The drawing under review shows one solid part. Ordinate dimensions are in mm from its lowest x, y, z. A direction names the side the tool comes from. Give positions to 0.01 mm unless a question says otherwise; leave off trailing zeros. Loops run counter-clockwise (first coordinate to the right, second up) from the corner with the lowest first, then second, coordinate; pieces in that order, holes last. Notation, with made-up numbers: (-4, 57.25) - (42, 57.25) arc R28 ccw to (42, 91.25) - close; hole circle Ø4 at (-10.5, -32.5). An arc over 180 degrees is marked (long way). Return JSON: item names as keys, results as strings. Group by question number.
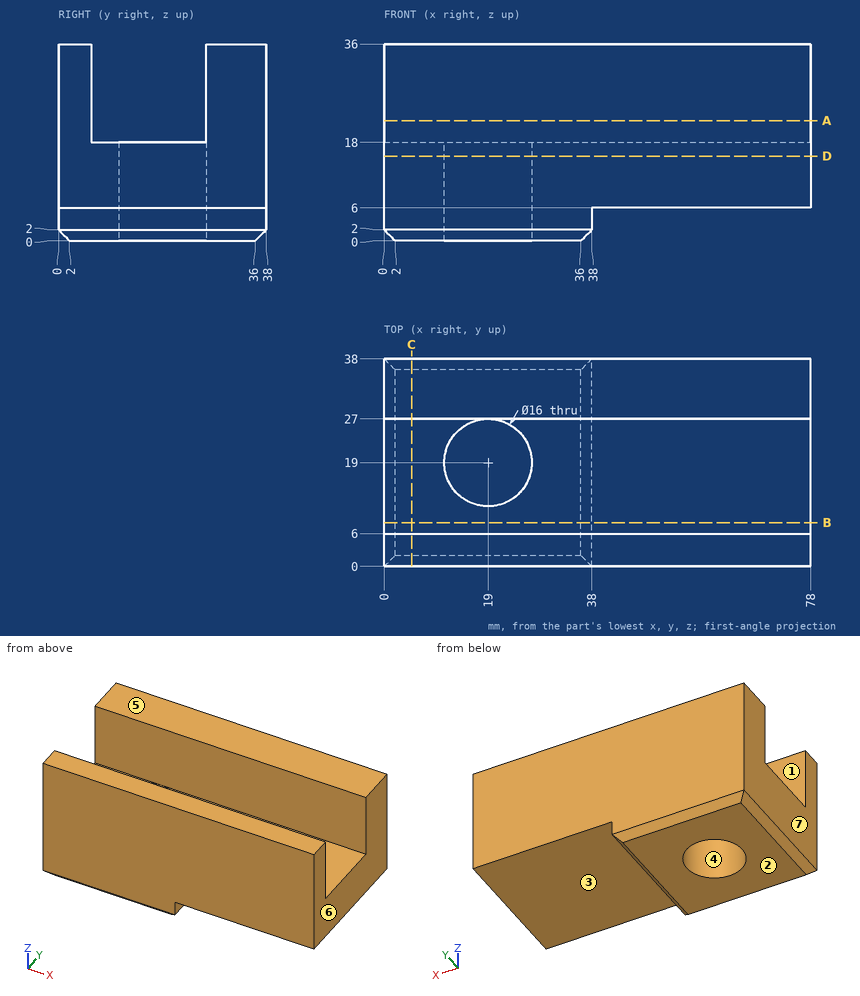
1) Draft analysis for pull direction X (two halves, no side actions). For the marked faces 4, 5, 6 and 7, state which applies: +X half, -X half, draft (parallel to the pull), parting line (faces both ways), or undercut.
2) We need section A-A, the plane z = 22. Write out the cut boundary in (x, y), plus the area to 3 significant figures.
3) Tool access review of the marked faces 1, 2 and 3: name each direction out of +Z, -Z, +X, -X, +Y, -Y from which nothing blocks a thin tool from reaching the whole face with its end or side.
4) For pin 1 Ø9.5 at (x, y) = (19, 19) entering from +Z; pin 2 Ø10.5 at (x, y) = (37.5, 18) entering from +Z; pin 3 Ø2 at (y, z) = (10.5, 4.5) entering from +X, all flat-tipped, find the tip position at first contact; note any pin that passes through.
5) We need section B-B, the plane y = 8. Write out the cut boundary in (x, z).
6) To check wall thickness, follow line 1 (X direction, y = 19, z = 3.5); line 2 (Y direction, x = 61.5, z = 21.5). State the ranges of each line that lie inside material, in increasing order.
7) We need section D-D, the plane z = 15.5. Write out the cut boundary in (x, y), plus the area to 3 significant figures.
8) We need section C-C, the plane x = 5. Write out the cut boundary in (y, z).
Findings:
{
 "1": {"face 4": "undercut", "face 5": "draft", "face 6": "+X half", "face 7": "-X half"},
 "2": {"outline": "(0, 0) - (78, 0) - (78, 6) - (0, 6) - close; (0, 27) - (78, 27) - (78, 38) - (0, 38) - close", "area": "1,330 mm^2"},
 "3": {"face 1": "+Z, +X, -X", "face 2": "-Z, +X, -X, +Y, -Y", "face 3": "-Z, +X, +Y, -Y"},
 "4": {"pin 1": "passes through", "pin 2": "stops at z = 18", "pin 3": "stops at x = 38"},
 "5": {"outline": "(0, 2) - (2, 0) - (36, 0) - (38, 2) - (38, 6) - (78, 6) - (78, 18) - (0, 18) - close"},
 "6": {"line 1": "x = 0 to 11, 27 to 38", "line 2": "y = 0 to 6, 27 to 38"},
 "7": {"outline": "(0, 0) - (78, 0) - (78, 38) - (0, 38) - close; hole circle Ø16 at (19, 19)", "area": "2,760 mm^2"},
 "8": {"outline": "(0, 2) - (2, 0) - (36, 0) - (38, 2) - (38, 36) - (27, 36) - (27, 18) - (6, 18) - (6, 36) - (0, 36) - close"}
}
